```python
from build123d import *

# Parameters (mm, degrees)
P_IDAT_VYSUNUT_M1_DEPTH  = 30
SKICA2_R                 = 12.5
ODEBRAT_VYSUNUT_M1_DEPTH = 30
SKICA3_R                 = 1.5
ODEBRAT_VYSUNUT_M2_DEPTH = 30


with BuildPart() as part:
    # Skica1 → Přidat vysunutím1 (new body)
    with BuildSketch(Plane(origin=(0, 0, 0), x_dir=(1, 0, 0), z_dir=(0, 1, 0))):
        with BuildLine():
            Line((-15, 2), (-15, 0))
            Line((-15, 0), (-15, -15))
            Line((-15, -15), (15, -15))
            Line((15, -15), (15, 0))
            Line((15, 0), (15, 2))
            Line((15, 2), (12.338962679, 2))
            ThreePointArc((12.338962679, 2), (12.459675628, 1.00323639), (12.5, 0))
            ThreePointArc((12.5, 0), (-1.00323639, -12.459675628), (-12.338962679, 2))
            Line((-12.338962679, 2), (-15, 2))
        make_face()
    extrude(amount=P_IDAT_VYSUNUT_M1_DEPTH)

    # Skica2 → Odebrat vysunutím1 (cut)
    with BuildSketch(Plane.XY.offset(15)):
        with Locations((0, 15)):
            Circle(SKICA2_R)
    extrude(amount=-ODEBRAT_VYSUNUT_M1_DEPTH, mode=Mode.SUBTRACT)

    # Skica3 → Odebrat vysunutím2 (cut)
    with BuildSketch(Plane.XY.offset(15)):
        with Locations((-12, 27)):
            Circle(SKICA3_R)
        with Locations((12, 27)):
            Circle(SKICA3_R)
        with Locations((12, 3)):
            Circle(SKICA3_R)
        with Locations((-12, 3)):
            Circle(SKICA3_R)
    extrude(amount=-ODEBRAT_VYSUNUT_M2_DEPTH, mode=Mode.SUBTRACT)


solid = part.part
```
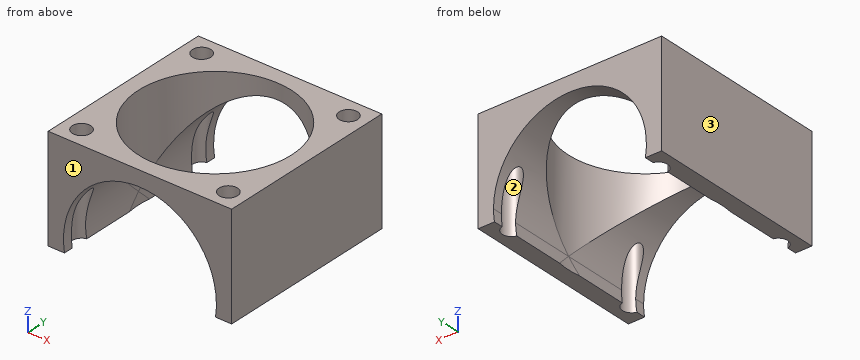
The model under review builds one solid part; all positions refer to its coordinate system, in mm. Face numbers are marked on the shaded views. Give positions to 0.01 mm unless a question says otherwise; leave off trailing zeros. Write each loop counter-clockwise with the first axis right and the second up, starting at its lowest first coordinate (ties: lowest second). Pieces come first, ordered by that corner, then holes. Notation, with made-up numbers: M 49.25,58 L 92.25,58 A24 ccw 92.25,94 Z; hole C 86.5,40.25 d2. An arc over 180 degrees is marked long. Answer in a Markdown table with one row per item.
Item 1: Add section D-D on y = 27. Give the boundary of the cut face in (x, z), plus the area to 3 significant figures.
Check sheet entries:
| item | result |
|---|---|
| outline | M -15,-2 L -13.5,-2 L -13.5,15 L -15,15 Z; M -10.5,6.78 A12.5 cw -3.5,12 L -3.5,15 L -10.5,15 Z; M 3.5,12 A12.5 cw 10.5,6.78 L 10.5,15 L 3.5,15 Z; M 13.5,-2 L 15,-2 L 15,15 L 13.5,15 Z |
| area | 120 mm2 |
Item 2: For line 1 along X through (y, z) = (27.5, 11); line 2 along Y through (x, z) = (13, 10.75); line 3 along Y through (x, z) = (-7.5, 10.75), list the stretches that pass through material, from the lowest coordinate up.
Check sheet entries:
| item | result |
|---|---|
| line 1 | -15 to -13.41, -10.59 to -5.94, 5.94 to 10.59, 13.41 to 15 |
| line 2 | 0 to 1.88, 4.12 to 25.88, 28.12 to 30 |
| line 3 | 0 to 5, 25 to 30 |
Item 3: Draft analysis for pull direction Y (two halves, no side actions). For the marked faces 1, 2 and 3, state which applies: +Y half, -Y half, draft (parallel to the pull), parting line (faces both ways), or undercut.
Check sheet entries:
| item | result |
|---|---|
| face 1 | -Y half |
| face 2 | undercut |
| face 3 | draft |
Item 4: Add section B-B on x = 0. Give the boundary of the cut face in (y, z), plus the area to 3 significant figures.
Check sheet entries:
| item | result |
|---|---|
| outline | M 0,12.5 L 2.5,12.5 L 2.5,15 L 0,15 Z; M 27.5,12.5 L 30,12.5 L 30,15 L 27.5,15 Z |
| area | 12.5 mm2 |
Item 5: For P1, Ø1.8, axis at x = 12, y = 27, coming from the +Z side, flat-tipped, find the tip position at first contact; note if it passes through.
Check sheet entries:
| item | result |
|---|---|
| P1 | through |
Item 6: Add section C-C on y = 8.5. Give the boundary of the cut face in (x, z).
Check sheet entries:
| item | result |
|---|---|
| outline | M -15,-2 L -12.34,-2 A12.5 cw -10.68,6.5 L -10.68,15 L -15,15 Z; M 10.68,6.5 A12.5 cw 12.34,-2 L 15,-2 L 15,15 L 10.68,15 Z |
Item 7: Add section A-A on z = 10.75. Give the boundary of the cut face in (x, y), plus the area to 3 significant figures.
Check sheet entries:
| item | result |
|---|---|
| outline | M -15,0 L -6.38,0 L -6.38,4.25 A12.5 cw -6.38,25.75 L -6.38,30 L -15,30 Z; M 6.38,0 L 15,0 L 15,30 L 6.38,30 L 6.38,25.75 A12.5 cw 6.38,4.25 Z; hole C -12,3 d3; hole C -12,27 d3; hole C 12,3 d3; hole C 12,27 d3 |
| area | 303 mm2 |
